Read the model definition and answer for the solid it produces. Units are mm, in the model's axes. Face numbers are marked on the shaded views. A direction names the side the tool comes from. Coordinates: 2 decimals unless noted, no trailing zeros. Loops run counter-clockwise (first coordinate to the right, second up) from the corner with the lowest first, then second, coordinate; pieces in that order, holes last. Notation, with made-up numbers: (78, 88) -> (83, 88) arc R22 ccw to (83, 114) -> close; hole circle Ø2 at (9, -25). An arc over 180 degrees is marked (long way). Answer as a JSON object with one key per item and string values. Group by question number.
Q1. The part is cut by section B-B on y = 91.5. Write down the section's boundary in (x, z), and give its area (3 significant figures).
Q2. Straight lines are drawn through the part: line 1 along X through (y, z) = (15, 0); line 2 along Y through (x, z) = (11.5, -14); line 3 along X through (y, z) = (42.5, 0). For each, find the intervals that lie inside material, in ascending order. Write a range as [from, to].
Q3. The part is cut by section A-A on y = 79. Write down the section's boundary in (x, z).
Q4. Each of these flat-tipped pins is pushed along its axis until it touches: P1, Ø21, axis at x = 4, z = -2.5, coming from the -Y side; P2, Ø2, axis at x = -16.5, y = 44.5, coming from the -Z side; P3, Ø12, axis at y = 23.5, z = -5, coming from the +X side; P4, Ø5, axis at y = 90.5, z = -17, coming from the -X side. Where does it stop, or does it pass through?
Q5. Determine the mould class of the marked faces 3, 4 and 5 for opening direction X: released by +X, released by -X, zero draft, split by the parting line, or undercut.
Q6. For the marked faces 1 and 2, determine the directions among +Z, -Z, +X, -X, +Y, -Y from which every point of the face is accessible in a straight line to the end or side of a thin tool.
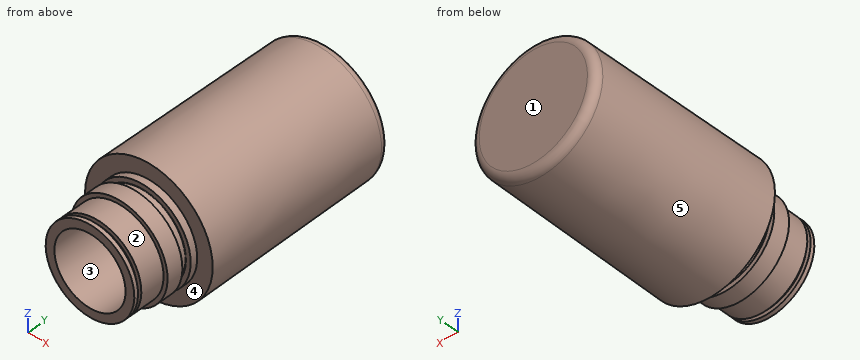
from build123d import *

# Parameters (mm, degrees)
FILLET2_R        = 3.175
FILLET4_R        = 0.127
HC843E_FILLET3_R = 3.175


with BuildPart() as part:
    # Sketch1 → Revolve1 (revolve)
    with BuildSketch(Plane.XY, mode=Mode.PRIVATE) as revolve1_sk:
        Polygon((-13.97, 0), (-17.399, 0), (-17.399, 1.5875), (-15.7607, 1.5875), (-15.7607, 3.0099), (-17.399, 3.0099), (-17.399, 12.5349), (-18.9738, 12.5349), (-18.9738, 18.8849), (-17.018, 18.8849), (-17.018, 22.4409), (-18.9738, 22.4409), (-18.9738, 25.2349), (-18.308812674, 101.4349), (0, 101.4349), (0, 96.3549), (-12.7, 96.3549), (-13.009873622, 60.8469), (-13.97, 60.8469), (-13.97, 60.0269), (-14.7, 60.0269), (-14.7, 58.7269026), (-13.97, 58.7269026), (-13.97, 37.9349), (-14.7, 37.9349), (-14.7, 36.6349026), (-13.97, 36.6349026), align=None)
    revolve(revolve1_sk.sketch.rotate(Axis((0, 0, 0), (0, 1, 0)), 270), axis=Axis((0, 0, 0), (0, 1, 0)))

    # Fillet2
    fillet2_edges = [part.edges().sort_by_distance(p)[0] for p in [
        (0, 96.3549, 12.7),
    ]]
    fillet(fillet2_edges, radius=FILLET2_R)

    # Fillet4
    fillet4_edges = [part.edges().sort_by_distance(p)[0] for p in [
        (0, 22.4409, 17.018),
        (0, 18.8849, 17.018),
    ]]
    fillet(fillet4_edges, radius=FILLET4_R)

    # Sketch4 → HC843E Revolve3 (revolve)
    with BuildSketch(Plane.XY, mode=Mode.PRIVATE) as hc843e_revolve3_sk:
        Polygon((-18.308812674, 101.4349), (-24.387019881, 101.4349), (-25.052007206, 25.2349), (-18.9738, 25.2349), align=None)
    revolve(hc843e_revolve3_sk.sketch.rotate(Axis((0, 0, 0), (0, 1, 0)), 90), axis=Axis((0, 0, 0), (0, 1, 0)))

    # HC843E Fillet3
    hc843e_fillet3_edges = [part.edges().sort_by_distance(p)[0] for p in [
        (0, 101.4349, -24.387019881),
    ]]
    fillet(hc843e_fillet3_edges, radius=HC843E_FILLET3_R)


solid = part.part
Final values:
{
 "1": {"outline": "circle Ø48.95 at (0, 0); hole circle Ø25.48 at (0, 0)", "area": "1,370 mm2"},
 "2": {"line 1": "x = [-18.97, -13.97], [13.97, 18.97]", "line 2": "y = [12.53, 18.88], [22.44, 101.43]", "line 3": "x = [-24.9, -13.97], [13.97, 24.9]"},
 "3": {"outline": "circle Ø49.17 at (0, 0); hole circle Ø25.7 at (0, 0)"},
 "4": {"P1": "stops at y = 0", "P2": "stops at z = -19.47", "P3": "stops at x = 25.05", "P4": "stops at x = -19.73"},
 "5": {"face 3": "undercut", "face 4": "zero draft", "face 5": "split by the parting line"},
 "6": {"face 1": "+Z, -Z, +X, -X, +Y", "face 2": "-Y"}
}
